Build history of the part. All positions in model axes, mm. Coordinates: 2 decimals unless noted, no trailing zeros. Order: outer loops, then holes, each group sorted by start corner. A loop starts at its lowest first (then second) coordinate and runs counter-clockwise, first axis right, second up. Notation, with made-up numbers: M 88,16.5 L 115,16.5 A10 ccw 115,30.5 Z; hole C 5.25,49 d9. An arc over 180 degrees is marked long. Write item = value, one per line. Start each with the question number.
Q1. Pin check, flat tips, straight feed: P1, Ø4, axis at x = 449.5, z = 1079, coming from the +Y side; P2, Ø4, axis at x = 402, z = 1076, coming from the +Y side. Stop position of each tip, or through.
Q2. Band-saw the part on C-C on x = 401. Write the cut outline in (y, z), plus the area to 3 significant figures.
Q3. Band-saw the part on A-A on y = 652.5. Write the cut outline in (x, z).
Q4. Band-saw the part on B-B on z = 1074.75. Write the cut outline in (x, y) (1 decimal), plus the area to 3 significant figures.
Q5. Drill centre lines: probe 1 along X at (y, z) = (347.5, 1077.25); probe 2 along X at (y, z) = (660, 1070); probe 3 along Y at (x, z) = (410, 1072.25). Where is each one in solid material? Low to high.
Q6. Band-saw the part on D-D on x = 178.5. Write the cut outline in (y, z), plus the area to 3 significant figures.
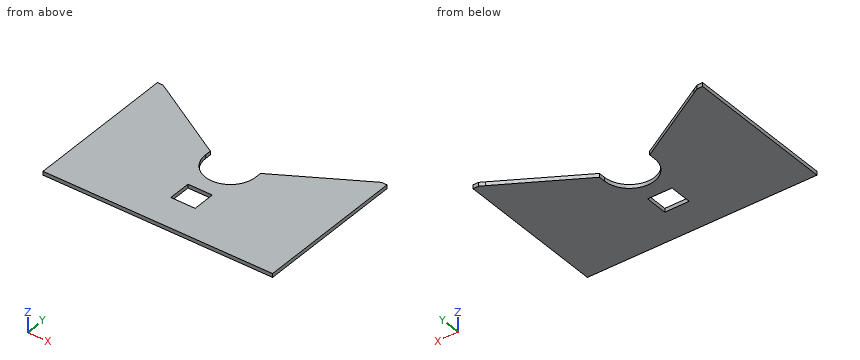
```python
from build123d import *

# Parameters (mm, degrees)
BOSS_EXTRUDE1_DEPTH = 12.7
SKETCH7_W           = 81.817014572
SKETCH7_H           = 76.120378059
CUT_EXTRUDE5_DEPTH  = 12.7


with BuildPart() as part:
    # Sketch1 → Boss-Extrude1 (new body)
    with BuildSketch(Plane.XY.offset(1081.90385267)):
        with BuildLine():
            Line((477.370001613, 579.113460481), (743.688832794, 732.872709354))
            Line((743.688832794, 732.872709354), (760.186616736, 742.397709354))
            Line((760.186616736, 742.397709354), (779.236616736, 742.397709354))
            Line((779.236616736, 742.397709354), (779.236616736, 234.397709354))
            Line((779.236616736, 234.397709354), (6.593386489, 234.397709354))
            Line((6.593386489, 234.397709354), (6.593386489, 742.397709354))
            Line((6.593386489, 742.397709354), (25.643386489, 742.397709354))
            Line((25.643386489, 742.397709354), (42.141170431, 732.872709354))
            Line((42.141170431, 732.872709354), (308.460001613, 579.113460481))
            Line((308.460001613, 579.113460481), (308.460001613, 557.307056284))
            ThreePointArc((308.460001613, 557.307056284), (392.915001613, 472.852056284), (477.370001613, 557.307056284))
            Line((477.370001613, 557.307056284), (477.370001613, 579.113460481))
        make_face()
    extrude(amount=-BOSS_EXTRUDE1_DEPTH)

    # Sketch7 → Cut-Extrude5 (cut)
    with BuildSketch(Plane(origin=(0, 0, 1069.20385267), x_dir=(-1, 0, 0), z_dir=(0, 0, -1))):
        with Locations((-392.915001613, 384.334045895)):
            Rectangle(SKETCH7_W, SKETCH7_H)
    extrude(amount=-CUT_EXTRUDE5_DEPTH, mode=Mode.SUBTRACT)


solid = part.part
```
Recorded:
q1.P1 = 496.48
q1.P2 = 473.58
q2.outline = M 234.4,1069.2 L 346.27,1069.2 L 346.27,1081.9 L 234.4,1081.9 Z; M 422.39,1069.2 L 473.24,1069.2 L 473.24,1081.9 L 422.39,1081.9 Z
q2.area = 2,070 mm2
q3.outline = M 6.59,1069.2 L 181.35,1069.2 L 181.35,1081.9 L 6.59,1081.9 Z; M 604.48,1069.2 L 779.24,1069.2 L 779.24,1081.9 L 604.48,1081.9 Z
q4.outline = M 6.6,234.4 L 779.2,234.4 L 779.2,742.4 L 760.2,742.4 L 477.4,579.1 L 477.4,557.3 A84.5 cw 308.5,557.3 L 308.5,579.1 L 25.6,742.4 L 6.6,742.4 Z; hole M 352,346.3 L 433.8,346.3 L 433.8,422.4 L 352,422.4 Z
q4.area = 298,000 mm2
q5.probe_1 = 6.59 to 352.01, 433.82 to 779.24
q5.probe_2 = 6.59 to 168.36, 617.47 to 779.24
q5.probe_3 = 234.4 to 346.27, 422.39 to 474.6
q6.outline = M 234.4,1069.2 L 654.15,1069.2 L 654.15,1081.9 L 234.4,1081.9 Z
q6.area = 5,330 mm2
